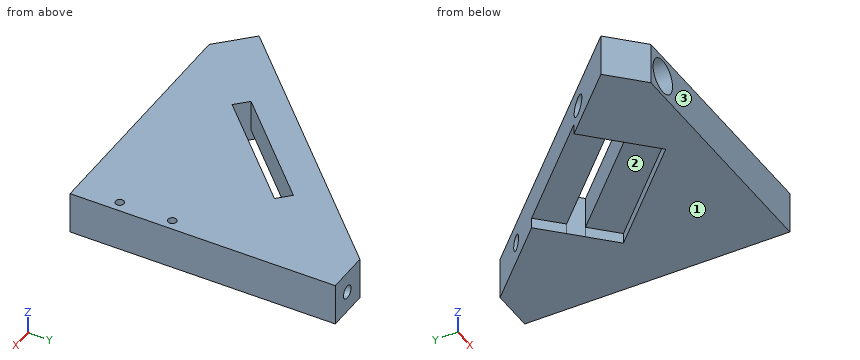
```python
from build123d import *

# Parameters (mm, degrees)
BOSS_EXTRUDE1_DEPTH            = 4
SKETCH3_W                      = 59.68
SKETCH3_H                      = 8
BOSS_EXTRUDE2_DEPTH            = 5.46
CUT_EXTRUDE1_DEPTH             = 9
SKETCH5_W                      = 59.68
SKETCH5_H                      = 2.16
CUT_EXTRUDE2_DEPTH             = 10
CUT_EXTRUDE7_DEPTH             = 10
M2X0_4_TAPPED_HOLE1_D          = 1.6
M2X0_4_TAPPED_HOLE1_DEPTH      = 7
M2X0_4_TAPPED_HOLE1_TIP        = 0.480688495
CBORE_FOR_M3_SHCS2_D           = 3.4
CBORE_FOR_M3_SHCS2_CBORE_D     = 6.5
CBORE_FOR_M3_SHCS2_CBORE_DEPTH = 3
CUT_EXTRUDE10_DEPTH            = 9
SKETCH24_R                     = 1.5
CUT_EXTRUDE12_DEPTH            = 5.5
M3X0_5_TAPPED_HOLE3_D          = 2.5
M3X0_5_TAPPED_HOLE3_DEPTH      = 8.5
M3X0_5_TAPPED_HOLE3_TIP        = 0.751075774
CUT_EXTRUDE13_DEPTH            = 2


with BuildPart() as part:
    # Sketch2 → Boss-Extrude1 (new body, symmetric)
    with BuildSketch(Plane.XY):
        Polygon((-8.360559535, 17.409242356), (51.319440465, 17.409242356), (51.319440465, 71.653558741), (36.009440465, 71.653558741), (43.084036895, 64.586021309), (-1.285963105, 20.171704924), (-8.360559535, 27.239242356), align=None)
    extrude(amount=BOSS_EXTRUDE1_DEPTH, both=True)

    # Sketch3 → Boss-Extrude2 (add)
    with BuildSketch(Plane.XZ.offset(-17.409242356)):
        with Locations((21.479440465, 0)):
            Rectangle(SKETCH3_W, SKETCH3_H)
    extrude(amount=BOSS_EXTRUDE2_DEPTH)

    # Sketch4 → Cut-Extrude1 (cut, through all)
    with BuildSketch(Plane(origin=(0, 0, -4), x_dir=(-1, 0, 0), z_dir=(0, 0, -1))):
        Polygon((-33.450754625, 46.445299472), (-35.748851663, 44.147202433), (-17.08123264, 25.47958341), (-14.783135601, 27.777680449), align=None)
    extrude(amount=-CUT_EXTRUDE1_DEPTH, mode=Mode.SUBTRACT)

    # Sketch5 → Cut-Extrude2 (cut)
    with BuildSketch(Plane(origin=(0, 0, -4), x_dir=(-1, 0, 0), z_dir=(0, 0, -1))):
        with Locations((-21.479440465, 13.029242356)):
            Rectangle(SKETCH5_W, SKETCH5_H)
    extrude(amount=-CUT_EXTRUDE2_DEPTH, mode=Mode.SUBTRACT)

    # Sketch7 → Cut-Extrude7 (cut)
    with BuildSketch(Plane(origin=(0, 0, -4), x_dir=(-1, 0, 0), z_dir=(0, 0, -1))):
        Polygon((1.285963105, 20.171704924), (-5.082290623, 13.803451195), (8.360559535, 13.803451195), (8.360559535, 14.109242356), (8.360559535, 29.043387574), (1.285963105, 29.043387574), align=None)
    extrude(amount=-CUT_EXTRUDE7_DEPTH, mode=Mode.SUBTRACT)

    # M2x0.4 Tapped Hole1
    with Locations(Plane.XY.offset(4)):
        with Locations((49.319440465, 32.429242356), (49.319440465, 22.429242356)):
            Hole(M2X0_4_TAPPED_HOLE1_D / 2, depth=M2X0_4_TAPPED_HOLE1_DEPTH)
            with Locations((0, 0, -(M2X0_4_TAPPED_HOLE1_DEPTH + M2X0_4_TAPPED_HOLE1_TIP / 2))):  # 118° drill point
                Cone(0, M2X0_4_TAPPED_HOLE1_D / 2, M2X0_4_TAPPED_HOLE1_TIP, mode=Mode.SUBTRACT)

    # CBORE for M3 SHCS2 (through all)
    with Locations(Plane(origin=(0, 14.109242356, 0), x_dir=(-1, 0, 0), z_dir=(0, -1, 0))):
        with Locations((-8.776499462, 0)):
            CounterBoreHole(CBORE_FOR_M3_SHCS2_D / 2, CBORE_FOR_M3_SHCS2_CBORE_D / 2, CBORE_FOR_M3_SHCS2_CBORE_DEPTH)

    # Sketch22 → Cut-Extrude10 (cut, through all)
    with BuildSketch(Plane(origin=(0, 0, -4), x_dir=(-1, 0, 0), z_dir=(0, 0, -1))):
        Polygon((-43.084036895, 64.586021309), (-51.319440465, 64.586021309), (-51.319440465, 71.653558741), (-36.009440465, 71.653558741), align=None)
    extrude(amount=-CUT_EXTRUDE10_DEPTH, mode=Mode.SUBTRACT)

    # Sketch24 → Cut-Extrude12 (cut)
    with BuildSketch(Plane(origin=(-10.729470873, 10.71876506, 0), x_dir=(0, 0, 1), z_dir=(-0.707459643, 0.706753743, 0))):
        with Locations((0, 66.141807925)):
            Circle(SKETCH24_R)
    extrude(amount=-CUT_EXTRUDE12_DEPTH, mode=Mode.SUBTRACT)

    # M3x0.5 Tapped Hole3
    with Locations(Plane(origin=(0, 64.586021309, 0), x_dir=(1, 0, 0), z_dir=(0, 1, 0))):
        with Locations((47.319440465, 0)):
            Hole(M3X0_5_TAPPED_HOLE3_D / 2, depth=M3X0_5_TAPPED_HOLE3_DEPTH)
            with Locations((0, 0, -(M3X0_5_TAPPED_HOLE3_DEPTH + M3X0_5_TAPPED_HOLE3_TIP / 2))):  # 118° drill point
                Cone(0, M3X0_5_TAPPED_HOLE3_D / 2, M3X0_5_TAPPED_HOLE3_TIP, mode=Mode.SUBTRACT)

    # Sketch28 → Cut-Extrude13 (cut)
    with BuildSketch(Plane(origin=(0, 0, -4), x_dir=(-1, 0, 0), z_dir=(0, 0, -1))):
        Polygon((-33.450754625, 46.445299472), (-35.748851663, 44.147202433), (-40.345045741, 39.551008355), (-21.677426718, 20.883389332), (-17.08123264, 25.47958341), (-14.783135601, 27.777680449), (-10.545665345, 32.015150705), (-29.20396649, 50.692087606), align=None)
    extrude(amount=-CUT_EXTRUDE13_DEPTH, mode=Mode.SUBTRACT)


solid = part.part
```
For this review, take the finished solid that the model builds, in its own axes (mm). Face numbers are marked on the shaded views. Round coordinates to 2 decimals unless told otherwise and drop trailing zeros. Write each loop counter-clockwise with the first axis right and the second up, starting at its lowest first coordinate (ties: lowest second). Pieces come first, ordered by that corner, then holes. Notation, with made-up numbers: (23.5, 6.5) - (60.5, 6.5) arc R18 ccw to (60.5, 15.5) - close; hole circle Ø8 at (23.25, -7.75). An arc over 180 degrees is marked (long way). Answer as CSV lines item,"result". Start each with the question number.
(1) Add section C-C, the plane y = 24. State the section outline as (x, z) points.
(2) Add section A-A, the plane y = 41. State the section outline as (x, z) points.
(3) Add section B-B, the plane z = 2.5. State the section outline as (x, y) points.
(4) For line 1 (X direction, y = 32, z = -0.25); line 2 (X direction, y = 27.5, z = -0.5); line 3 (X direction, y = 26, z = 3.5), list the stretches that pass through material, from the lowest coordinate up.
(5) For pin 1 (8 mm diameter, centred on x = 16.5, y = 35, fed in from -Z); pin 2 (12 mm diameter, centred on x = 7.5, y = 39.5, fed in from -Z); pin 3 (12 mm diameter, centred on x = 8.5, y = 31.5, fed in from +Z); pin 4 (4 mm diameter, centred on x = 8.78, z = 0, fed in from +Y), all flat-tipped, find the tip position at first contact; note any pin that passes through.
(6) Mouldability with a two-part tool opening along Y and no side actions: class the marked faces 1, 2 and 3 as +Y half, -Y half, draft (parallel to the pull), parting line (faces both ways), or undercut.
From the geometry:
1,outline,"(2.54, -4) - (18.56, -4) - (18.56, -2) - (24.79, -2) - (24.79, -4) - (51.32, -4) - (51.32, 4) - (2.54, 4) - close; hole circle Ø3.4 at (8.78, 0)"
2,outline,"(19.52, -2) - (28.01, -2) - (28.01, 4) - (19.52, 4) - close; (32.6, -2) - (38.9, -2) - (38.9, -4) - (51.32, -4) - (51.32, 4) - (32.6, 4) - close"
3,outline,"(-1.29, 20.17) - (4.78, 14.11) - (6.7, 14.11) - (6.7, 17.11) - (10.85, 17.11) - (10.85, 14.11) - (51.32, 14.11) - (51.32, 64.59) - (43.08, 64.59) - close; hole (14.78, 27.78) - (17.08, 25.48) - (35.75, 44.15) - (33.45, 46.45) - close; hole circle Ø1.6 at (49.32, 22.43); hole circle Ø1.6 at (49.32, 32.43)"
4,line 1,"x = 10.53 to 19.01, 23.6 to 48.64, 49.99 to 51.32"
4,line 2,"x = 6.04 to 7.15, 10.4 to 15.06, 19.1 to 51.32"
4,line 3,"x = 4.54 to 16.56, 17.6 to 51.32"
5,pin 1,"stops at z = -2"
5,pin 2,"passes through"
5,pin 3,"stops at z = 4"
5,pin 4,"stops at y = 32.25"
6,face 1,"draft"
6,face 2,"undercut"
6,face 3,"-Y half"
